from build123d import *

# Parameters (mm, degrees)
SKETCH1_W           = 23.83
SKETCH1_H           = 1
BOSS_EXTRUDE1_DEPTH = 22.5
SKETCH2_R           = 1.325
BOSS_EXTRUDE2_DEPTH = 14.25
BOSS_EXTRUDE4_DEPTH = 8
SKETCH5_W           = 21.979847568
SKETCH5_H           = 2.5
BOSS_EXTRUDE5_DEPTH = 40
SKETCH6_R           = 4.25
SKETCH6_R_2         = 1.05
CUT_EXTRUDE1_DEPTH  = 76.367433285
FILLET1_R           = 7
FILLET2_R           = 7
FILLET3_R           = 7
BOSS_EXTRUDE6_START = 41
BOSS_EXTRUDE6_DEPTH = 41


with BuildPart() as part:
    # Sketch1 → Boss-Extrude1 (new body)
    with BuildSketch(Plane(origin=(0, 0, 0), x_dir=(1, 0, 0), z_dir=(0, 1, 0))):
        Rectangle(SKETCH1_W, SKETCH1_H)
    extrude(amount=BOSS_EXTRUDE1_DEPTH)

    # Sketch2 → Boss-Extrude2 (add, symmetric)
    with BuildSketch(Plane(origin=(0, 11.25, 0), x_dir=(1, 0, 0), z_dir=(0, 1, 0))):
        with Locations(Location((-11.915, 0, 0), (0, 0, 270))):
            Circle(SKETCH2_R)
        with Locations(Location((11.915, 0, 0), (0, 0, 270))):
            Circle(SKETCH2_R)
    extrude(amount=BOSS_EXTRUDE2_DEPTH, both=True)

    # Sketch4 → Boss-Extrude4 (add, symmetric)
    with BuildSketch(Plane(origin=(0, 0, 0), x_dir=(0, 0, -1), z_dir=(1, 0, 0))):
        Polygon((-0.5, 19.001100744), (-0.5, 22.5), (-12.5, 34.25), (-35.5, 34.25), (-35.5, 31.75), (-13.520152432, 31.75), align=None)
        Polygon((-0.5, 0), (-0.5, 3.498899256), (-13.520152432, -9.25), (-35.5, -9.25), (-35.5, -11.75), (-12.5, -11.75), align=None)
    extrude(amount=BOSS_EXTRUDE4_DEPTH, both=True)

    # Sketch5 → Boss-Extrude5 (add)
    with BuildSketch(Plane.ZY.offset(8)):
        with Locations((24.510076216, 33)):
            Rectangle(SKETCH5_W, SKETCH5_H)
        with Locations((24.510076216, -10.5)):
            Rectangle(SKETCH5_W, SKETCH5_H)
    extrude(amount=BOSS_EXTRUDE5_DEPTH)

    # Sketch6 → Cut-Extrude1 (cut, through all)
    with BuildSketch(Plane(origin=(0, 34.25, 0), x_dir=(1, 0, 0), z_dir=(0, 1, 0))):
        with Locations(Location((-37.010076216, -24.510076216, 0), (0, 0, 270))):
            Circle(SKETCH6_R)
        with Locations(Location((-44.010076216, -24.510076216, 0), (0, 0, 270))):
            Circle(SKETCH6_R_2)
        with Locations(Location((-37.010076216, -17.510076216, 0), (0, 0, 270))):
            Circle(SKETCH6_R_2)
        with Locations(Location((-30.010076216, -24.510076216, 0), (0, 0, 270))):
            Circle(SKETCH6_R_2)
        with Locations(Location((-37.010076216, -31.510076216, 0), (0, 0, 270))):
            Circle(SKETCH6_R_2)
        with BuildLine():
            ThreePointArc((-48, -24.510076216), (-44.781125848, -16.739026584), (-37.010076216, -13.520152432))
            Line((-37.010076216, -13.520152432), (-48, -13.520152432))
            Line((-48, -13.520152432), (-48, -24.510076216))
        make_face()
        with BuildLine():
            ThreePointArc((-37.010076216, -35.5), (-44.781125848, -32.281125848), (-48, -24.510076216))
            Line((-48, -24.510076216), (-48, -35.5))
            Line((-48, -35.5), (-37.010076216, -35.5))
        make_face()
    extrude(amount=-CUT_EXTRUDE1_DEPTH, mode=Mode.SUBTRACT)

    # Fillet1
    # the kernel refuses this fillet: 7 mm, written as the material it adds along each edge
    with BuildSketch(Plane(origin=(-8, -11.75, 13.520152432), x_dir=(-1, 0, 0), z_dir=(0, 1, 0))) as fillet1_piece_1_section:
        with BuildLine():
            CenterArc((FILLET1_R, -FILLET1_R), FILLET1_R, 90, 90)
            Line((0, -FILLET1_R), (0, 0))
            Line((0, 0), (FILLET1_R, 0))
        make_face()
    fillet1_piece_1 = extrude(amount=2.5, mode=Mode.PRIVATE)
    fillet1_piece_1 = split(fillet1_piece_1, bisect_by=Plane(origin=(-10.011124011, -11.168341556, 11.905965844), z_dir=(0, 0.7145104264934944, 0.699624792608213)), keep=Keep.TOP, mode=Mode.PRIVATE)
    fillet1_piece_1 = split(fillet1_piece_1, bisect_by=Plane(origin=(-10.011124011, -9.382065489, 13.655027826), z_dir=(0, -0.7145104264934944, -0.6996247926082129)), keep=Keep.TOP, mode=Mode.PRIVATE)
    add(fillet1_piece_1)
    with BuildSketch(Plane(origin=(-8, -11.75, 13.520152432), x_dir=(-1, 0, 0), z_dir=(0, 1, 0))) as fillet1_piece_2_section:
        with BuildLine():
            CenterArc((FILLET1_R, -FILLET1_R), FILLET1_R, 90, 90)
            Line((0, -FILLET1_R), (0, 0))
            Line((0, 0), (FILLET1_R, 0))
        make_face()
    fillet1_piece_2 = extrude(amount=20, mode=Mode.PRIVATE)
    fillet1_piece_2 = split(fillet1_piece_2, bisect_by=Plane(origin=(-8.808469458, -8.892227761, 9.581424097), z_dir=(0, 0.7145104264934944, 0.699624792608213)), keep=Keep.TOP, mode=Mode.PRIVATE)
    fillet1_piece_2 = split(fillet1_piece_2, bisect_by=Plane(origin=(-8.808469458, -9.25, 10.72673952), z_dir=(0, 1, 0)), keep=Keep.TOP, mode=Mode.PRIVATE)
    fillet1_piece_2 = split(fillet1_piece_2, bisect_by=Plane(origin=(-8.808469458, -7.105951695, 11.330486078), z_dir=(0, -0.7145104264934944, -0.6996247926082129)), keep=Keep.TOP, mode=Mode.PRIVATE)
    add(fillet1_piece_2)
    with BuildSketch(Plane(origin=(-8, 34.25, 13.520152432), x_dir=(0, 0, -1), z_dir=(0, -1, 0))) as fillet1_piece_3_section:
        with BuildLine():
            CenterArc((FILLET1_R, -FILLET1_R), FILLET1_R, 90, 90)
            Line((0, -FILLET1_R), (0, 0))
            Line((0, 0), (FILLET1_R, 0))
        make_face()
    fillet1_piece_3 = extrude(amount=2.5, mode=Mode.PRIVATE)
    fillet1_piece_3 = split(fillet1_piece_3, bisect_by=Plane(origin=(-10.011124011, 31.882065489, 13.655027826), z_dir=(0, 0.7145104264934944, -0.6996247926082129)), keep=Keep.TOP, mode=Mode.PRIVATE)
    fillet1_piece_3 = split(fillet1_piece_3, bisect_by=Plane(origin=(-10.011124011, 33.668341556, 11.905965844), z_dir=(0, -0.7145104264934944, 0.699624792608213)), keep=Keep.TOP, mode=Mode.PRIVATE)
    add(fillet1_piece_3)
    with BuildSketch(Plane(origin=(-8, 34.25, 13.520152432), x_dir=(0, 0, -1), z_dir=(0, -1, 0))) as fillet1_piece_4_section:
        with BuildLine():
            CenterArc((FILLET1_R, -FILLET1_R), FILLET1_R, 90, 90)
            Line((0, -FILLET1_R), (0, 0))
            Line((0, 0), (FILLET1_R, 0))
        make_face()
    fillet1_piece_4 = extrude(amount=20, mode=Mode.PRIVATE)
    fillet1_piece_4 = split(fillet1_piece_4, bisect_by=Plane(origin=(-8.808469465, 29.605951697, 11.33048608), z_dir=(0, 0.7145104264934944, -0.6996247926082129)), keep=Keep.TOP, mode=Mode.PRIVATE)
    fillet1_piece_4 = split(fillet1_piece_4, bisect_by=Plane(origin=(-8.808469465, 31.392227764, 9.581424099), z_dir=(0, -0.7145104264934944, 0.699624792608213)), keep=Keep.TOP, mode=Mode.PRIVATE)
    fillet1_piece_4 = split(fillet1_piece_4, bisect_by=Plane(origin=(-8.808469465, 31.75, 10.726739522), z_dir=(0, -1, 0)), keep=Keep.TOP, mode=Mode.PRIVATE)
    add(fillet1_piece_4)
    # the kernel refuses this fillet: 7 mm, written as the material it takes off along each edge
    with BuildSketch(Plane(origin=(8, 8.25, 35.5), x_dir=(0, 0, -1), z_dir=(0, -1, 0))) as fillet1_2_piece_1:
        with BuildLine():
            CenterArc((FILLET1_R, -FILLET1_R), FILLET1_R, 90, 90)
            Line((0, -FILLET1_R), (0, 0))
            Line((0, 0), (FILLET1_R, 0))
        make_face()
    extrude(amount=37.5, mode=Mode.SUBTRACT)
    with BuildSketch(Plane(origin=(8, 51.75, 35.5), x_dir=(-1, 0, 0), z_dir=(0, -1, 0))) as fillet1_2_piece_2:
        with BuildLine():
            CenterArc((FILLET1_R, FILLET1_R), FILLET1_R, 180, 90)
            Line((0, FILLET1_R), (0, 0))
            Line((0, 0), (FILLET1_R, 0))
        make_face()
    extrude(amount=37.5, mode=Mode.SUBTRACT)

    # Fillet2
    fillet2_edges = [part.edges().sort_by_distance(p)[0] for p in [
        (0, 19.001100744, 0.5),
        (0, 3.498899256, 0.5),
    ]]
    fillet(fillet2_edges, radius=FILLET2_R)

    # Fillet3
    # the kernel refuses this fillet: 7 mm, written as the material it adds along each edge
    with BuildSketch(Plane(origin=(-8, 22.5, 0.5), x_dir=(0, 0.6996247926074847, 0.7145104264942074), z_dir=(1, 0, 0))) as fillet3_piece_1:
        with BuildLine():
            CenterArc((2.335944006, -7), FILLET3_R, 90, 25.834886249)
            Line((-0.714510426, -0.699624793), (0, 0))
            Line((0, 0), (2.335944006, 0))
        make_face()
    extrude(amount=16)
    with BuildSketch(Plane(origin=(8, 0, 0.5), x_dir=(0, 0, -1), z_dir=(-1, 0, 0))) as fillet3_piece_2:
        with BuildLine():
            CenterArc((3.2283172, 6.635857326), FILLET3_R, 225.603091194, 25.834886249)
            Line((-1.669056348, 1.634284341), (0, 0))
            Line((0, 0), (1, 0))
        make_face()
    extrude(amount=16)

    # Sketch8 → Boss-Extrude6 (add)
    with BuildSketch(Plane(origin=(0, -9.25, 0), x_dir=(1, 0, 0), z_dir=(0, 1, 0)).offset(BOSS_EXTRUDE6_START)):
        with BuildLine():
            ThreePointArc((1, -35.5), (5.949747468, -33.449747468), (8, -28.5))
            Line((8, -28.5), (5, -28.5))
            ThreePointArc((5, -28.5), (3.422054899, -30.922054899), (1, -32.5))
            Line((1, -32.5), (1, -35.5))
        make_face()
    extrude(amount=-BOSS_EXTRUDE6_DEPTH)


solid = part.part
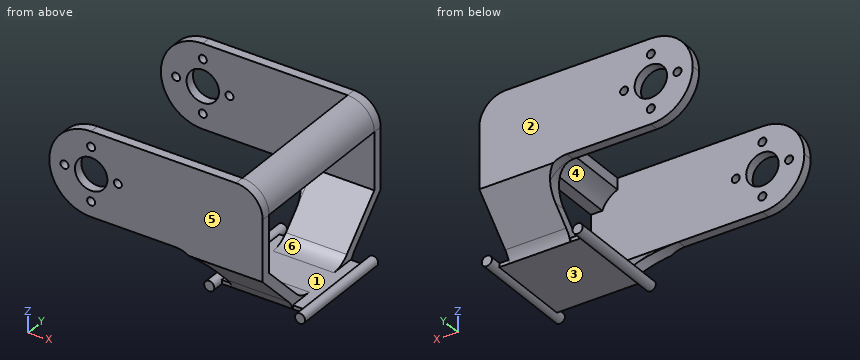
CAD build for the part. Positions are in the model's coordinates, mm. Face numbers are marked on the shaded views. A direction names the side the tool comes from. Give positions to 0.01 mm unless a question says otherwise; leave off trailing zeros. Loops run counter-clockwise (first coordinate to the right, second up) from the corner with the lowest first, then second, coordinate; pieces in that order, holes last. Notation, with made-up numbers: M 82.25,82 L 103.25,82 A22 cw 103.25,120 Z; hole C 0,58.5 d10. An arc over 180 degrees is marked long. One line per question, with ' | ' between items. Start each with the question number.
1. Saw through at B-B on y = 14. Give the cut face in (x, z) (3 decimals).
2. Flat gauge pins, fed straight in: pin 1 (0.8 mm diameter, centred on x = 12.5, z = 0, fed in from -Y); pin 2 (8 mm diameter, centred on y = 2, z = 13, fed in from -X); pin 3 (0.5 mm diameter, centred on x = -9, z = 0, fed in from -Y); pin 4 (3 mm diameter, centred on x = -24.5, y = 33.5, fed in from -Z). Where does each tip first touch, or does it go through?
3. Probe L1, parallel to Y at x = -32.5, z = 20; L2, parallel to Z at x = -9, y = 4.5; L3, parallel to Y at x = 3.5, z = 4. List the from-to ranges inside material, lowest first. Write a range as from..to.
4. Saw through at D-D on z = 27. Give the cut face in (x, y).
5. Saw through at A-A on x = -21.5. Give the cut face in (y, z), plus the area to 3 significant figures.
6. 3-axis set-ups, long thin cutter, end or side, ignore diameter. For the marked faces 1 and 2: which of +Z, -Z, +X, -X, +Y, -Y reach the whole face in a straight line?
7. Two-plate mould, pull along Y, no slides. Class the marked faces 3, 4, 5 and 6: pulls with the +Y half, pulls with the -Y half, needs draft (parallel to the pull), parting line crosses it, or undercut.
8. Saw through at C-C on x = -1. Give the cut face in (y, z).
Result sheet:
1) outline: M -10.688,-0.5 L 10.688,-0.5 A1.325 ccw long 10.688,0.5 L -10.688,0.5 A1.325 ccw long Z; M 1,32.5 A7 cw 5,28.5 L 8,28.5 A7 ccw 1,35.5 Z
2) pin 1: stops at y = -3 | pin 2: passes through | pin 3: stops at y = 0 | pin 4: stops at z = 13.52
3) L1: y = -11.75..-9.25, 31.75..34.25 | L2: z = -0.5..0.5 | L3: y = -3.43..0.07, 22.43..25.93
4) outline: M -47.71,-11.75 L -40.45,-11.75 L -40.45,-9.25 L -47.71,-9.25 Z; M -47.71,31.75 L -40.45,31.75 L -40.45,34.25 L -47.71,34.25 Z; M -33.57,-11.75 L 8,-11.75 L 8,-9.25 L -33.57,-9.25 Z; M -33.57,31.75 L 8,31.75 L 8,34.25 L -33.57,34.25 Z
5) outline: M -11.75,13.52 L -9.25,13.52 L -9.25,35.5 L -11.75,35.5 Z; M 31.75,13.52 L 34.25,13.52 L 34.25,35.5 L 31.75,35.5 Z | area: 110 mm^2
6) face 1: none | face 2: +Z, -Z, +X, -X, +Y
7) face 3: needs draft | face 4: undercut | face 5: pulls with the -Y half | face 6: undercut
8) outline: M -11.75,12.5 L -1.63,2.17 A7 cw 0,-0.5 L 22.5,-0.5 A7 cw 24.13,2.17 L 34.25,12.5 L 34.25,35.5 L 31.75,35.5 L 31.75,13.52 L 21.06,2.6 A7 cw 16.06,0.5 L 6.44,0.5 A7 cw 1.44,2.6 L -9.25,13.52 L -9.25,35.5 L -11.75,35.5 Z
